Print and shaded views of the part. All mm, measured from the part's lowest x, y and z. Round coordinates to 2 decimals unless told otherwise and drop trailing zeros. Loops run counter-clockwise (first coordinate to the right, second up) from the corner with the lowest first, then second, coordinate; pieces in that order, holes last. Notation, with made-up numbers: (89.5, 75) -> (133.5, 75) arc R26 cw to (133.5, 93) -> close; hole circle Ø6 at (2, 6.5). An arc over 180 degrees is marked (long way). Use a Markdown table: item, result.
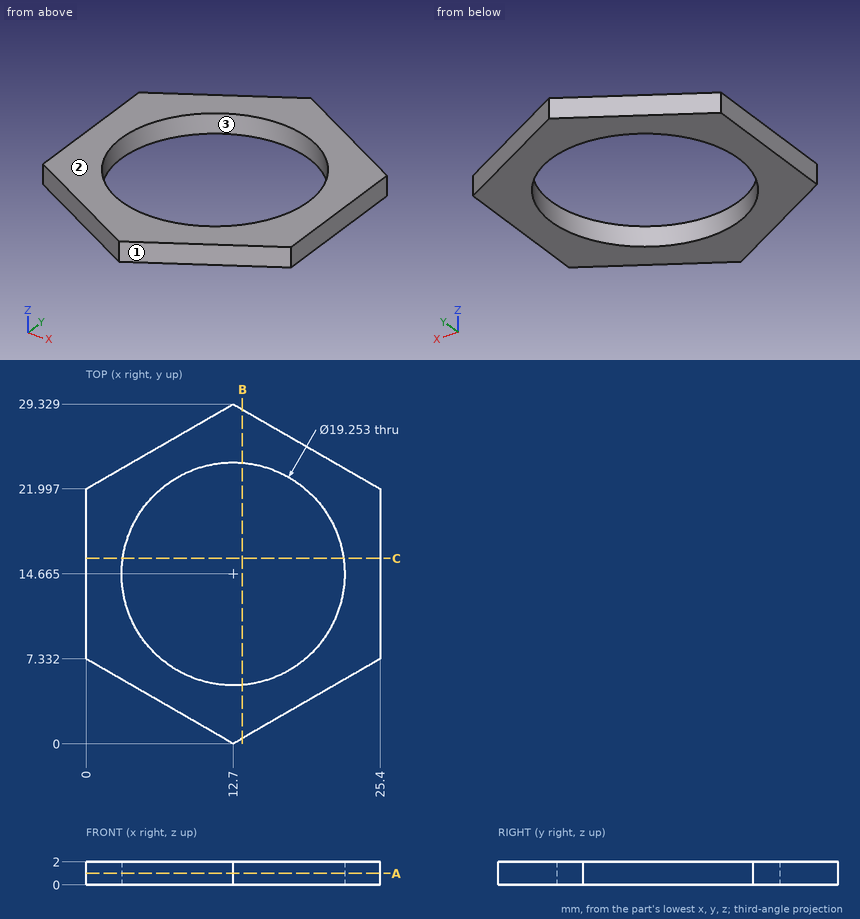
Q1. Band-saw the part on C-C, the plane y = 16. Give the cut face in (x, z).
Results list:
| item | result |
|---|---|
| outline | (0, 0) -> (3.17, 0) -> (3.17, 2) -> (0, 2) -> close; (22.23, 0) -> (25.4, 0) -> (25.4, 2) -> (22.23, 2) -> close |
Q2. Band-saw the part on B-B, the plane x = 13.5. Give the cut face in (y, z).
Results list:
| item | result |
|---|---|
| outline | (0.46, 0) -> (5.07, 0) -> (5.07, 2) -> (0.46, 2) -> close; (24.26, 0) -> (28.87, 0) -> (28.87, 2) -> (24.26, 2) -> close |
Q3. Drill centre lines: L1, parallel to X at y = 10, z = 0.7; L2, parallel to X at y = 11.5, z = 1.25; L3, parallel to Y at x = 9.5, z = 0.3 (1 decimal). Where is each one in solid material? Low to high. Write a range as from..to.
Results list:
| item | result |
|---|---|
| L1 | x = 0..4.28, 21.12..25.4 |
| L2 | x = 0..3.61, 21.79..25.4 |
| L3 | y = 1.8..5.6, 23.7..27.5 |
Q4. Band-saw the part on A-A, the plane z = 1. Give the cut face in (x, y) (1 decimal).
Results list:
| item | result |
|---|---|
| outline | (0, 7.3) -> (12.7, 0) -> (25.4, 7.3) -> (25.4, 22) -> (12.7, 29.3) -> (0, 22) -> close; hole circle Ø19.3 at (12.7, 14.7) |
Q5. Pull direction Y, two halves, no side cores. Call the marked faces 1, 2 and 3: released by +Y, released by -Y, zero draft, split by the parting line, or undercut.
Results list:
| item | result |
|---|---|
| face 1 | released by -Y |
| face 2 | zero draft |
| face 3 | undercut |
